Answer from the drawing. Dimensions are ordinates in mm from the lowest x, y and z of the part. A direction names the side the tool comes from. Give positions to 0.01 mm unless a question says otherwise; leave off trailing zeros. Loops run counter-clockwise (first coordinate to the right, second up) from the corner with the lowest first, then second, coordinate; pieces in that order, holes last.
(1) Straight lines are drawn through the part: probe 1 along Z at (x, y) = (59.4, 61.5); probe 2 along X at (y, z) = (68.5, 5.75); probe 3 along X at (y, z) = (36, 1.25). For each, find the intervals that lie inside material, in ascending order.
(2) Find section A-A, the plane y = 18.5. Write down the section's boundary in (x, z).
(3) Find section C-C, the plane x = 10. Write down the section's boundary in (y, z), then the cut area to 3 significant figures.
(4) Find section D-D, the plane y = 60. Write down the section's boundary in (x, z), then the cut area to 3 significant figures.
(5) Find section B-B, the plane z = 4. Write down the section's boundary in (x, y), then the cut area to 3 significant figures.
(6) Which of the six approach directions +Z, -Z, +X, -X, +Y, -Y give full straight-line access (tool end or side, diameter ignored) to the marked faces 1 and 2?
(7) Each of these flat-tipped pins is pushed along its axis until it touches: P1, Ø4.5, axis at y = 61.5, z = 3.944, coming from the +X side; P2, Ø0.8, axis at x = 1.5, z = 5, coming from the -Y side; P3, Ø2.5, axis at x = 21, z = 4, coming from the -Y side. Where does it stop, or does it pass through?
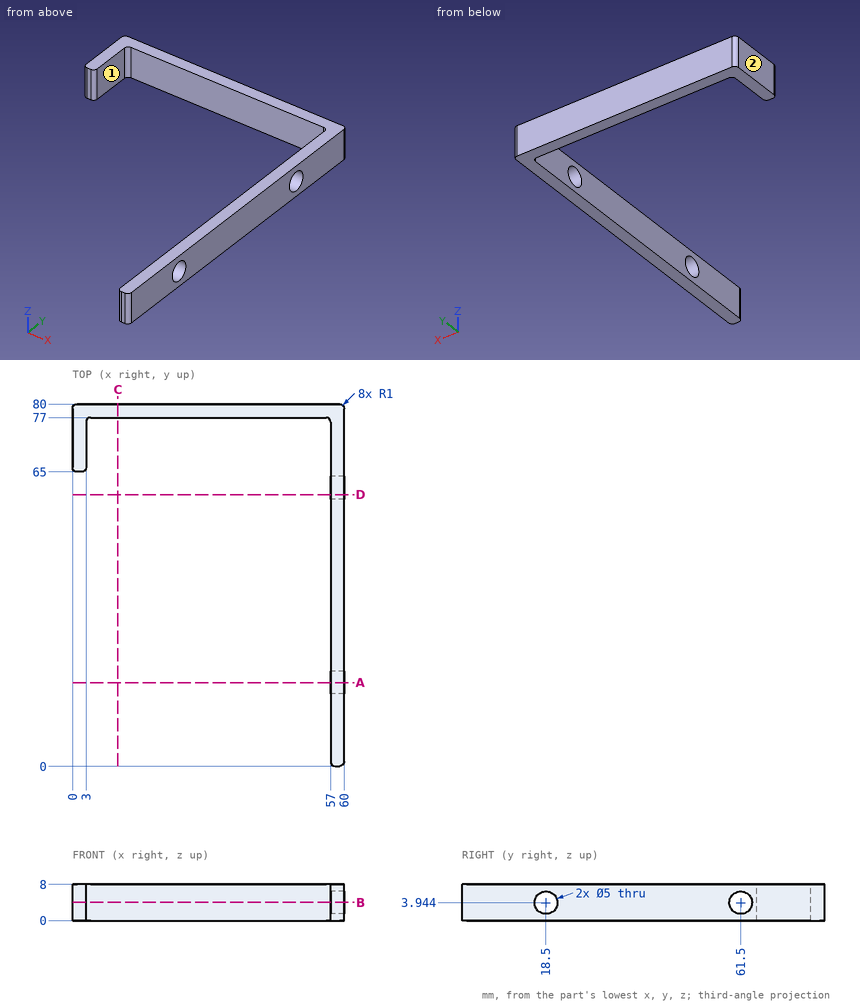
Entries:
1. probe 1: z = 0 to 1.44, 6.44 to 8
1. probe 2: x = 0 to 3, 57 to 60
1. probe 3: x = 57 to 60
2. outline: (57, 0) - (60, 0) - (60, 1.44) - (57, 1.44) - close; (57, 6.44) - (60, 6.44) - (60, 8) - (57, 8) - close
3. outline: (77, 0) - (80, 0) - (80, 8) - (77, 8) - close
3. area: 24.0 mm2
4. outline: (57, 0) - (60, 0) - (60, 1.94) - (57, 1.94) - close; (57, 5.94) - (60, 5.94) - (60, 8) - (57, 8) - close
4. area: 12.0 mm2
5. outline: (0, 66) arc R1 ccw to (1, 65) - (2, 65) arc R1 ccw to (3, 66) - (3, 76) arc R1 cw to (4, 77) - (56, 77) arc R1 cw to (57, 76) - (57, 64) - (60, 64) - (60, 79) arc R1 ccw to (59, 80) - (1, 80) arc R1 ccw to (0, 79) - close; (57, 1) arc R1 ccw to (58, 0) - (59, 0) arc R1 ccw to (60, 1) - (60, 16) - (57, 16) - close; (57, 21) - (60, 21) - (60, 59) - (57, 59) - close
5. area: 416 mm2
6. face 1: +Z, -Z, -Y
6. face 2: +Z, -Z, -X, +Y, -Y
7. P1: passes through
7. P2: stops at y = 65
7. P3: stops at y = 77
